For this review, take the finished solid that the model builds, in its own axes (mm). Face numbers are marked on the shaded views. A direction names the side the tool comes from. Coordinates: 2 decimals unless noted, no trailing zeros. Loops run counter-clockwise (first coordinate to the right, second up) from the corner with the lowest first, then second, coordinate; pieces in that order, holes last. Notation, with made-up numbers: (64, 87.5) -> (100, 87.5) arc R16 ccw to (100, 102.5) -> close; hole circle Ø9 at (26.25, -15.75). An arc over 180 degrees is marked (long way). One line per item, written item: value.
from build123d import *

# Parameters (mm, degrees)
SKETCH1_W           = 13
SKETCH1_H           = 2
SKETCH1_W_2         = 2
SKETCH1_H_2         = 37
SKETCH1_W_3         = 18
BOSS_EXTRUDE1_DEPTH = 40
SKETCH2_R           = 1.5
CUT_EXTRUDE1_DEPTH  = 40
FILLET1_R           = 1
SKETCH4_R           = 1.5
CUT_EXTRUDE2_DEPTH  = 40


with BuildPart() as part:
    # Sketch1 → Boss-Extrude1 (new body)
    with BuildSketch(Plane(origin=(0, 0, 0), x_dir=(0, 0, -1), z_dir=(1, 0, 0))):
        with Locations((6.5, 1)):
            Rectangle(SKETCH1_W, SKETCH1_H)
        with Locations((14, 1)):
            Rectangle(SKETCH1_W_2, SKETCH1_H)
        with Locations((14, -18.5)):
            Rectangle(SKETCH1_W_2, SKETCH1_H_2)
        with Locations((24, -38)):
            Rectangle(SKETCH1_W_3, SKETCH1_H)
        with Locations((14, -38)):
            Rectangle(SKETCH1_W_2, SKETCH1_H)
    extrude(amount=BOSS_EXTRUDE1_DEPTH)

    # Sketch2 → Cut-Extrude1 (cut)
    with BuildSketch(Plane(origin=(0, 2, 0), x_dir=(1, 0, 0), z_dir=(0, 1, 0))):
        with Locations(Location((10, 5, 0), (0, 0, 270))):
            Circle(SKETCH2_R)
        with Locations(Location((30, 5, 0), (0, 0, 270))):
            Circle(SKETCH2_R)
    extrude(amount=-CUT_EXTRUDE1_DEPTH, mode=Mode.SUBTRACT)

    # Fillet1
    fillet1_edges = [part.edges().sort_by_distance(p)[0] for p in [
        (20, 2, -15),
        (20, -37, -15),
        (20, -39, -13),
        (20, 0, -13),
    ]]
    fillet(fillet1_edges, radius=FILLET1_R)

    # Sketch4 → Cut-Extrude2 (cut)
    with BuildSketch(Plane(origin=(0, -37, 0), x_dir=(1, 0, 0), z_dir=(0, 1, 0))):
        with Locations(Location((30, 23, 0), (0, 0, 270))):
            Circle(SKETCH4_R)
        with Locations(Location((10, 23, 0), (0, 0, 270))):
            Circle(SKETCH4_R)
    extrude(amount=-CUT_EXTRUDE2_DEPTH, mode=Mode.SUBTRACT)


solid = part.part
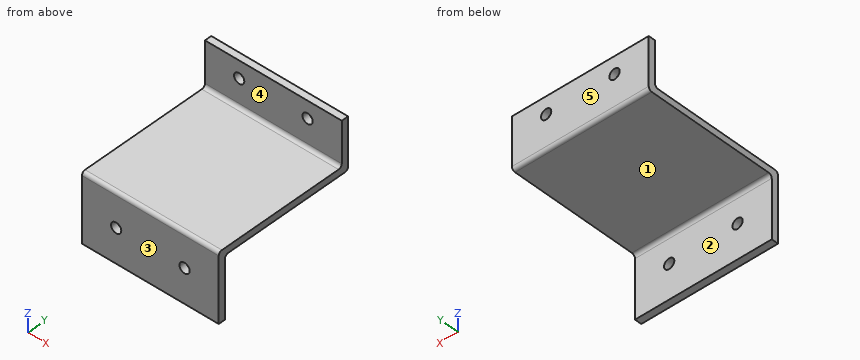
1. Take a section at B-B, the plane z = -23. Give the boundary of the cut face in (x, y).
Return value:
outline: (0, -39) -> (8.5, -39) -> (8.5, -37) -> (0, -37) -> close; (11.5, -39) -> (28.5, -39) -> (28.5, -37) -> (11.5, -37) -> close; (31.5, -39) -> (40, -39) -> (40, -37) -> (31.5, -37) -> close
2. Take a section at D-D, the plane z = -9.5. Give the boundary of the cut face in (x, y), and give its area (3 significant figures).
Return value:
outline: (0, 0) -> (40, 0) -> (40, 2) -> (0, 2) -> close
area: 80.0 mm2
3. To check wall thickness, follow probe 1 along X at (y, z) = (-38.2, -23); probe 2 along Y at (x, z) = (3.5, -3.5); probe 3 along Z at (x, y) = (11, -4). State the ranges of each line that lie inside material, in increasing order. Write a range as from..to.
Return value:
probe 1: x = 0..8.5, 11.5..28.5, 31.5..40
probe 2: y = 0..2
probe 3: z = -15..-13
4. The part is to be moulded in two halves that separate along Y. For the marked faces 1, 2 and 3, say which applies: pulls with the +Y half, pulls with the -Y half, needs draft (parallel to the pull), parting line crosses it, or undercut.
Return value:
face 1: needs draft
face 2: pulls with the +Y half
face 3: pulls with the -Y half
5. Insertion check: pin 1 Ø4 at (x, z) = (10, -5) entering from +Y; pin 2 Ø3.5 at (x, z) = (14, -4) entering from -Y; pin 3 Ø6 at (x, z) = (23.5, -19) entering from +Y; pin 4 Ø8 at (x, y) = (17, -29) entering from +Z. Each pin has a flat end and moves straight along its axis. Give the tip position at first contact, or say it passes through.
Return value:
pin 1: stops at y = 2
pin 2: stops at y = 0
pin 3: stops at y = -37
pin 4: stops at z = -13
6. Take a section at C-C, the plane x = 16. Give the boundary of the cut face in (y, z), and give its area (3 significant figures).
Return value:
outline: (-39, -33) -> (-37, -33) -> (-37, -16) arc R1 cw to (-36, -15) -> (1, -15) arc R1 ccw to (2, -14) -> (2, 0) -> (0, 0) -> (0, -12) arc R1 cw to (-1, -13) -> (-38, -13) arc R1 ccw to (-39, -14) -> close
area: 144 mm2
7. Take a section at A-A, the plane x = 30. Give the boundary of the cut face in (y, z), and give its area (3 significant figures).
Return value:
outline: (-39, -33) -> (-37, -33) -> (-37, -24.5) -> (-39, -24.5) -> close; (-39, -21.5) -> (-37, -21.5) -> (-37, -16) arc R1 cw to (-36, -15) -> (1, -15) arc R1 ccw to (2, -14) -> (2, -6.5) -> (0, -6.5) -> (0, -12) arc R1 cw to (-1, -13) -> (-38, -13) arc R1 ccw to (-39, -14) -> close; (0, -3.5) -> (2, -3.5) -> (2, 0) -> (0, 0) -> close
area: 132 mm2
8. For the marked faces 4 and 5, list the 3-axis set-ups (+Z, -Z, +X, -X, +Y, -Y) from which the entire face can be reached by the end or side of a thin tool; tool diameter is ignored.
Return value:
face 4: +Z, +X, -X, -Y
face 5: +Z, -Z, +X, -X, +Y
